Could you check a few things on this model? Use its own coordinates, in mm. A direction names the side the tool comes from. Coordinates: 2 decimals unless noted, no trailing zeros. Loops run counter-clockwise (first coordinate to the right, second up) from the corner with the lowest first, then second, coordinate; pieces in that order, holes last.
1) Imagine slicing it at A-A on y = 28.02. Please give me the cut outline in (x, z), plus the area to 3 significant figures.
2) Imagine slicing it at B-B on y = 22. Please give me the cut outline in (x, z), plus the area to 3 significant figures.
3) Imagine slicing it at D-D on x = 12.75. Please give me the cut outline in (y, z), plus the area to 3 significant figures.
4) Thinking about a two-plate mould opening in Z: for faces 1 (the face through (14.77, 20, -114)), 2 (the face through (8, 20, -118.92)), 3 (the face through (3, 15, -99.1)), 4 (the face through (3, 15, -81.8)), which applies, released by +Z, released by -Z, zero draft, split by the parting line, or undercut?
5) If I drill on line 1 along Y through (x, z) = (0.75, -5); line 2 along Z through (x, y) = (6.75, 27); line 3 along Y through (x, z) = (3.5, -99), over which ranges is the centre line in solid material (lowest first)?
6) Will these pins go through, and if not, where does the flat tip stop? P1, Ø4, axis at y = 4.5, z = -98.5, coming from the -X side; P2, Ø3.5, axis at x = 4.5, y = 15.5, coming from the -Z side; P3, Ø2, axis at y = 16.5, z = -71, coming from the +X side; P4, Ø4, axis at x = 5.5, z = -40.5, coming from the -Y side.
7) Imagine slicing it at C-C on x = 2.75. Give the number of separate pieces and of enclosed holes in the cut face, plus the area to 4 significant figures.
8) For faces 5 (the face through (3, 18.3, -7)), 6 (the face through (5.57, 15, -20)), 7 (the face through (3, 12, -97)), which set-ups out of +Z, -Z, +X, -X, +Y, -Y let a thin tool reach every point of the face, with its end or its side?
```python
from build123d import *

# Parameters (mm, degrees)
SKETCH1_W           = 121.92
SKETCH1_H           = 33.02
SKETCH1_R           = 1.5
BOSS_EXTRUDE1_DEPTH = 1.27
SKETCH2_W           = 9
SKETCH2_H           = 25.3
BOSS_EXTRUDE2_DEPTH = 13.5
SKETCH3_W           = 4.5
SKETCH3_H           = 6.3
BOSS_EXTRUDE3_DEPTH = 4.3


with BuildPart() as part:
    # Sketch1 → Boss-Extrude1 (new body)
    with BuildSketch(Plane(origin=(0, 0, 0), x_dir=(0, 0, -1), z_dir=(1, 0, 0))):
        with Locations((60.96, 16.51)):
            Rectangle(SKETCH1_W, SKETCH1_H)
        with Locations((5, 28.02)):
            Circle(SKETCH1_R, mode=Mode.SUBTRACT)
    extrude(amount=BOSS_EXTRUDE1_DEPTH)

    # Sketch2 → Boss-Extrude2 (add)
    with BuildSketch(Plane(origin=(1.27, 0, 0), x_dir=(0, 0, -1), z_dir=(1, 0, 0))):
        with Locations((114.42, 19.87)):
            Rectangle(SKETCH2_W, SKETCH2_H)
    extrude(amount=BOSS_EXTRUDE2_DEPTH)

    # Sketch3 → Boss-Extrude3 (add)
    with BuildSketch(Plane(origin=(1.27, 0, 0), x_dir=(0, 0, -1), z_dir=(1, 0, 0))):
        with Locations((7.25, 15.15)):
            Rectangle(SKETCH3_W, SKETCH3_H)
        with Locations((20.05, 15.15)):
            Rectangle(SKETCH3_W, SKETCH3_H)
        with Locations((32.85, 15.15)):
            Rectangle(SKETCH3_W, SKETCH3_H)
        with Locations((45.65, 15.15)):
            Rectangle(SKETCH3_W, SKETCH3_H)
        with Locations((58.45, 15.15)):
            Rectangle(SKETCH3_W, SKETCH3_H)
        with Locations((71.25, 15.15)):
            Rectangle(SKETCH3_W, SKETCH3_H)
        with Locations((84.05, 15.15)):
            Rectangle(SKETCH3_W, SKETCH3_H)
        with Locations((96.85, 15.15)):
            Rectangle(SKETCH3_W, SKETCH3_H)
    extrude(amount=BOSS_EXTRUDE3_DEPTH)


solid = part.part
```
Filled in:
1. outline: (0, -121.92) - (1.27, -121.92) - (1.27, -118.92) - (14.77, -118.92) - (14.77, -109.92) - (1.27, -109.92) - (1.27, -6.5) - (0, -6.5) - close; (0, -3.5) - (1.27, -3.5) - (1.27, 0) - (0, 0) - close
1. area: 273 mm2
2. outline: (0, -121.92) - (1.27, -121.92) - (1.27, -118.92) - (14.77, -118.92) - (14.77, -109.92) - (1.27, -109.92) - (1.27, 0) - (0, 0) - close
2. area: 276 mm2
3. outline: (7.22, -118.92) - (32.52, -118.92) - (32.52, -109.92) - (7.22, -109.92) - close
3. area: 228 mm2
4. face 1: zero draft
4. face 2: released by -Z
4. face 3: undercut
4. face 4: undercut
5. line 1: y = 0 to 26.52, 29.52 to 33.02
5. line 2: z = -118.92 to -109.92
5. line 3: y = 12 to 18.3
6. P1: stops at x = 0
6. P2: stops at z = -118.92
6. P3: stops at x = 5.57
6. P4: passes through
7. separate pieces: 9
7. enclosed holes: 0
7. area: 454.5 mm2
8. face 5: +Z, +X, +Y
8. face 6: +Z, +X, +Y, -Y
8. face 7: +Z, +X, -Y
